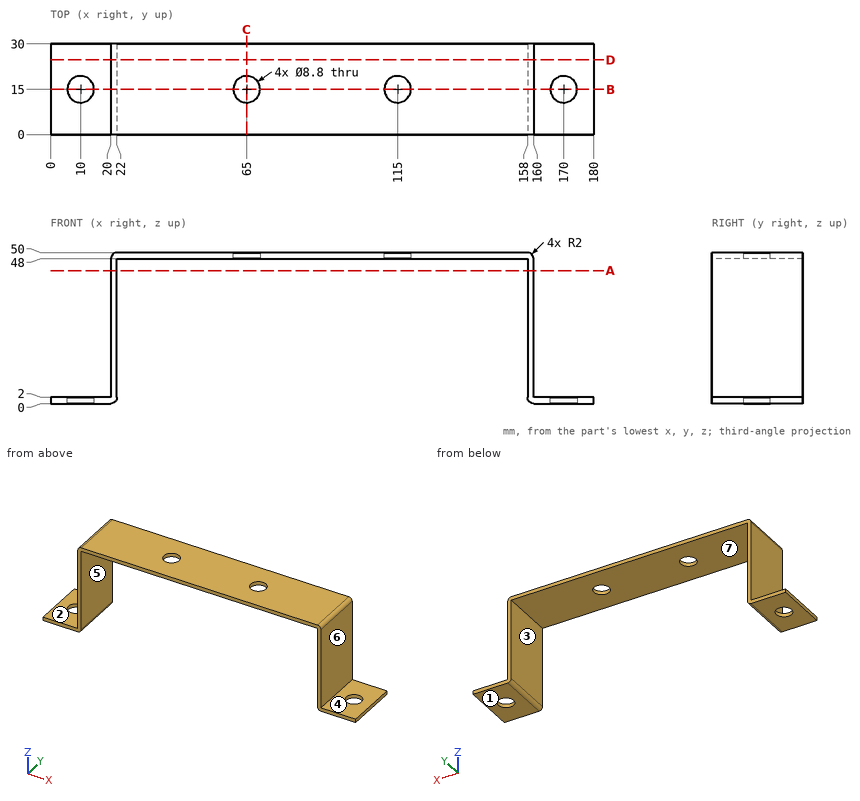
Verification items for this drawing (mm, ordinates from the low corner). A direction names the side the tool comes from. Coordinates: 2 decimals unless noted, no trailing zeros. Loops run counter-clockwise (first coordinate to the right, second up) from the corner with the lowest first, then second, coordinate; pieces in that order, holes last. Notation, with made-up numbers: (-37, 32) - (-6, 32) arc R20 ccw to (-6, 36) - close; hole circle Ø8 at (42.5, 0.5). An arc over 180 degrees is marked (long way). One line per item, written item: value. Start each with the question number.
(1) Cross-section at B-B on y = 15. Count the separate pieces of the cut face and the enclosed holes in it, plus the area to 3 significant figures.
(2) Material ranges on line 1 (X direction, y = 14.25, z = 6); line 2 (Y direction, x = 65, z = 49.4); line 3 (Z direction, x = 59.5, y = 12), recorded low to high. Write a range as [from, to].
(3) Depth check by flat-ended pin: P1, Ø7, axis at x = 65, y = 15, coming from the +Z side; P2, Ø1.5, axis at y = 25, z = 31, coming from the -X side; P3, Ø4, axis at x = 47, y = 21.5, coming from the -Z side; P4, Ø6, axis at y = 10, z = 11.5, coming from the +X side. Enter the tip coordinate at first touch or a pass-through.
(4) Cross-section at A-A on z = 44. Enter the section's corners in (x, y).
(5) Tool access check on the marked faces 1, 2 and 3. Record the directions out of +Z, -Z, +X, -X, +Y, -Y that give a thin tool (end or side, any length) a straight path to the whole face; none if there is none.
(6) Mould release check, pull along X, two halves, no side actions. Record for the marked faces 4, 5, 6 and 7: released by +X, released by -X, zero draft, split by the parting line, or undercut.
(7) Cross-section at D-D on y = 24.75. Enter the section's corners in (x, z), plus the area to 3 significant figures.
(8) Cross-section at C-C on x = 65. Enter the section's corners in (y, z).
Results below:
1. separate pieces: 5
1. enclosed holes: 0
1. area: 478 mm2
2. line 1: x = [20, 22], [158, 160]
2. line 2: y = [0, 10.6], [19.4, 30]
2. line 3: z = [48, 50]
3. P1: passes through
3. P2: stops at x = 20
3. P3: stops at z = 48
3. P4: stops at x = 160
4. outline: (20, 0) - (22, 0) - (22, 30) - (20, 30) - close; (158, 0) - (160, 0) - (160, 30) - (158, 30) - close
5. face 1: -Z, +X, -X, +Y, -Y
5. face 2: +Z, -X, +Y, -Y
5. face 3: -Z, +Y, -Y
6. face 4: zero draft
6. face 5: undercut
6. face 6: released by +X
6. face 7: undercut
7. outline: (0, 0) - (20, 0) arc R2 ccw to (22, 2) - (22, 48) - (158, 48) - (158, 2) arc R2 ccw to (160, 0) - (180, 0) - (180, 2) - (160, 2) - (160, 48) arc R2 ccw to (158, 50) - (22, 50) arc R2 ccw to (20, 48) - (20, 2) - (0, 2) - close
7. area: 549 mm2
8. outline: (0, 48) - (10.6, 48) - (10.6, 50) - (0, 50) - close; (19.4, 48) - (30, 48) - (30, 50) - (19.4, 50) - close
